Autodesk Inventor part; units mm, degrees
ref_plane "Plano de trabajo2" through (-10, 0, 0) normal (1, 0, 0) x (0, 1, 0)
ref_plane "XZ Plane" through (0, 0, 0) normal (0, 1, 0) x (-1, 0, 0)
ref_plane "XY Plane" through (0, 0, 0) normal (0, 0, 1) x (1, 0, 0)
sketch "Boceto1" plane through (0, 0, 0) normal (0, 1, 0) x (-1, 0, 0)
  line L0 (10, 7.5) -> (-10, 7.5)
  line L1 (-10, 7.5) -> (-10, -7.5)
  line L2 (-10, -7.5) -> (10, -7.5)
  line L3 (10, -7.5) -> (10, 7.5)
  arc A0 (6, -7.5) -> (6, 7.5) centre (0.9688, 0) ccw
  arc A1 (-6, 7.5) -> (-6, -7.5) centre (-0.9688, 0) ccw
  point P0 (0, 0)
  point P1 (-10, 0)
  point P2 (0, -7.5)
  dimension "d0" = 20
  dimension "d1" = 15
  dimension "d2" = 4
  dimension "d3" = 4
  dimension "d4" = 4
  dimension "d5" = 4
extrude "Extrusión1" add sketch "Boceto1" along normal blind 25 contours A0 L2 A1 L0
sketch "Boceto2" plane through (0, 25, 0) normal (0, 1, 0) x (1, 0, 0)
  line L0 (-6, -7.5) -> (6, -7.5)
  arc A0 (6, -7.5) -> (6, 7.5) centre (0.9688, 0) ccw
  line L1 (6, 7.5) -> (-6, 7.5)
  arc A1 (-6, 7.5) -> (-6, -7.5) centre (-0.9688, 0) ccw
  arc A2 (4, -3) -> (-4, -3) centre (0, 0) ccw
  line L2 (0, 0) -> (0, -3)
  line L3 (0, -3) -> (-4, -3)
  line L4 (0, -3) -> (4, -3)
  dimension "d8" = 10
  dimension "d9" = 3
extrude "Extrusión2" add sketch "Boceto2" along normal blind 2 contours L4 L3 A2
sketch "Boceto3" plane through (0, 27, 0) normal (0, 1, 0) x (1, 0, 0)
  line L0 (-4, -3) -> (4, -3)
  arc A0 (4, -3) -> (-4, -3) centre (0, 0) ccw
  circle A1 centre (0, 0) radius 1
  dimension "d12" = 2
extrude "Extrusión3" add sketch "Boceto3" along normal blind 7 contours A1
sketch "Boceto4" plane through (-6, 0, 7.5) normal (0, 0, 1) x (1, 0, 0)
  line L0 (0, 0) -> (12, 0)
  line L1 (12, 0) -> (12, 25)
  line L2 (0, 25) -> (12, 25)
  line L3 (0, 0) -> (0, 25)
  line L4 (4, 8) -> (8, 8)
  line L5 (8, 8) -> (8, 4)
  line L6 (8, 4) -> (4, 4)
  line L7 (4, 4) -> (4, 8)
  arc A0 (10, 20) -> (10, 16) centre (10, 18) ccw
  line L8 (10, 20) -> (10, 16) construction
  line L9 (10, 20) -> (14, 20) construction
  arc A1 (2, 16) -> (2, 20) centre (2, 18) ccw
  line L10 (2, 20) -> (2, 16) construction
  line L11 (2, 20) -> (6, 20) construction
  line L12 (10, 20) -> (10, 16)
  line L13 (2, 16) -> (2, 20)
  point P0 (6, 0)
  point P1 (6, 4)
  point P2 (6, 0)
  dimension "d15" = 4
  dimension "d16" = 4
  dimension "d17" = 8
  dimension "d18" = 4
  dimension "d19" = 90
  dimension "d20" = 2
  dimension "d21" = 20
  dimension "d22" = 2
  dimension "d23" = 4
  dimension "d24" = 90
  dimension "d25" = 2
  dimension "d26" = 20
  dimension "d27" = 2
extrude "Extrusión4" cut sketch "Boceto4" against normal blind 1 contours L12 A0 | L13 A1
extrude "Extrusión5" cut sketch "Boceto4" against normal blind 8 contours L4 L5 L6 L7
ref_plane "Plano de trabajo1" through (10, 0, 0) normal (1, 0, 0) x (0, 1, 0)
sketch "Boceto5" plane through (10, 0, 0) normal (1, 0, 0) x (0, 1, 0)
  line L0 (0, 7.5) -> (0, -7.5)
  line L1 (0, -7.5) -> (25, -7.5)
  line L2 (25, 7.5) -> (25, -7.5)
  line L3 (0, 7.5) -> (25, 7.5)
  arc A0 (10, 5.5) -> (10, 1.5) centre (10, 3.5) ccw
  line L4 (10, 5.5) -> (10, 1.5)
  arc A1 (10, -1.5) -> (10, -5.5) centre (10, -3.5) ccw
  line L5 (10, -5.5) -> (10, -1.5)
  point P0 (0, 0)
  dimension "d32" = 4
  dimension "d33" = 2
  dimension "d34" = 10
  dimension "d35" = 2
  dimension "d36" = 4
  dimension "d37" = 2
  dimension "d38" = 10
  dimension "d39" = 2
extrude "Extrusión6" cut sketch "Boceto5" against normal blind 2 contours L4 A0 | L5 A1
ref_plane "Plano de trabajo2" through (-10, 0, 0) normal (1, 0, 0) x (0, 1, 0)
sketch "Boceto6" plane through (-10, 0, 0) normal (1, 0, 0) x (0, 1, 0)
  line L0 (0, -7.5) -> (0, 7.5)
  line L1 (0, 7.5) -> (25, 7.5)
  line L2 (25, -7.5) -> (25, 7.5)
  line L3 (0, -7.5) -> (25, -7.5)
  arc A0 (10, -1.5) -> (10, -5.5) centre (10, -3.5) ccw
  line L4 (10, -1.5) -> (10, -5.5)
  line L5 (10, -5.5) -> (10, -1.5)
  arc A1 (10, 5.5) -> (10, 1.5) centre (10, 3.5) ccw
  line L6 (10, 5.5) -> (10, 1.5)
  line L7 (10, 5.5) -> (10, 1.5)
  point P0 (0, 0)
extrude "Extrusión7" cut sketch "Boceto6" along normal blind 2 contours L4 A0 | L6 A1
sketch "Boceto7" plane through (0, 0, 0) normal (0, -1, 0) x (1, 0, 0)
  line L0 (-6, 7.5) -> (6, 7.5)
  arc A0 (-6, 7.5) -> (-6, -7.5) centre (-0.9688, 0) ccw
  line L1 (6, -7.5) -> (-6, -7.5)
  arc A1 (6, -7.5) -> (6, 7.5) centre (0.9688, 0) ccw
  circle A2 centre (0, 0) radius 2
  dimension "d44" = 4
extrude "Extrusión8" add sketch "Boceto7" along normal blind 1.75 contours A2
sketch "Boceto8" plane through (0, -1.75, 0) normal (0, -1, 0) x (1, 0, 0)
  circle A0 centre (0, 0) radius 2
  circle A1 centre (0, 0) radius 1
extrude "Extrusión9" add sketch "Boceto8" along normal blind 0.5 contours A1
properties part number "Motor" material "Aluminio 6061-O"
Work out the finished part from the listing and answer in its coordinate system (mm). A direction names the side the tool comes from. Give positions to 0.01 mm unless a question says otherwise; leave off trailing zeros. Loops run counter-clockwise (first coordinate to the right, second up) from the corner with the lowest first, then second, coordinate; pieces in that order, holes last. Notation, with made-up numbers: M -6,0.5 L 11,0.5 A24 cw 11,24.5 Z; hole C 57.25,-4 d9. An arc over 180 degrees is marked long. One line per item, written item: value. Start each with the question number.
1. Which of the six approach directions +Z, -Z, +X, -X, +Y, -Y give full straight-line access (tool end or side, diameter ignored) to faces 4 (the face through (8, 9, -3)), 5 (the face through (-8, 9, 4)), 6 (the face through (1, -1.75, -1)), 7 (the face through (0, 26, -5))?
2. Each of these flat-tipped pins is pushed along its axis until it touches: P1, Ø1.1, axis at y = 17.5, z = 7, coming from the -X side; P2, Ø4, axis at y = 25.5, z = -5, coming from the -X side; P3, Ø2, axis at x = -9, z = -2.5, coming from the -Y side. Where does it stop, or does it pass through?
3. Find section C-C (x = 0). Give the vertices of the cut face in (y, z).
4. Find section B-B (y = 18). Give the vertices of the cut face in (x, z), and give its area (3 significant figures).
5. Find section D-D (z = -2.5). Give the vertices of the cut face in (x, y).
6. Find section A-A (z = 0). Give the vertices of the cut face in (x, y).
7. Determine the mould class of faces 1 (the face through (-2, 6, 4)), 2 (the face through (0, -2, 1)), 3 (the face through (0, 34, 0)) for opening direction Y: released by +Y, released by -Y, zero draft, split by the parting line, or undercut.
8. Find the intervals of material crossed by probe 1 along Y at (x, z) = (-1.5, 4.25); probe 2 along Y at (x, z) = (-8, -1); probe 3 along X at (y, z) = (7, 3.75), in increasing order.
Reported:
1. face 4: +X
1. face 5: -X
1. face 6: -Y
1. face 7: +Y
2. P1: stops at x = -7.29
2. P2: stops at x = -9.46
2. P3: stops at y = 0
3. outline: M -2.25,-1 L -1.75,-1 L -1.75,-2 L 0,-2 L 0,-7.5 L 25,-7.5 L 25,-5 L 27,-5 L 27,-1 L 34,-1 L 34,1 L 27,1 L 27,3 L 25,3 L 25,7.5 L 8,7.5 L 8,-0.5 L 4,-0.5 L 4,7.5 L 0,7.5 L 0,2 L -1.75,2 L -1.75,1 L -2.25,1 Z
4. outline: M -6,-7.5 L 6,-7.5 A9.03 ccw 6,7.5 L 4,7.5 L 4,6.5 L 2,6.5 L 2,7.5 L -2,7.5 L -2,6.5 L -4,6.5 L -4,7.5 L -6,7.5 A9.03 ccw Z
4. area: 260 mm²
5. outline: M -9.65,0 L 9.65,0 L 9.65,8.27 L 8,8.27 L 8,10 L 9.65,10 L 9.65,25 L 4.33,25 L 4.33,27 L -4.33,27 L -4.33,25 L -9.65,25 L -9.65,10 L -8,10 L -8,8.27 L -9.65,8.27 Z
6. outline: M -10,0 L -2,0 L -2,-1.75 L -1,-1.75 L -1,-2.25 L 1,-2.25 L 1,-1.75 L 2,-1.75 L 2,0 L 10,0 L 10,25 L 5,25 L 5,27 L 1,27 L 1,34 L -1,34 L -1,27 L -5,27 L -5,25 L -10,25 Z; hole M -2,4 L 2,4 L 2,8 L -2,8 Z
7. face 1: undercut
7. face 2: zero draft
7. face 3: released by +Y
8. probe 1: y = 0 to 4, 8 to 25
8. probe 2: y = 0 to 25
8. probe 3: x = -9.18 to -2, 2 to 9.18
